Check sheet for the modelled part. Datum: model origin and axes. Units: mm. Face numbers are marked on the shaded views. A direction names the side the tool comes from. Round coordinates to 2 decimals unless told otherwise and drop trailing zeros. Write each loop counter-clockwise with the first axis right and the second up, starting at its lowest first coordinate (ties: lowest second). Pieces come first, ordered by that corner, then holes.
Item 1: Depth check by flat-ended pin: pin 1 (8.5 mm diameter, centred on x = -20, z = -13.5, fed in from -Y); pin 2 (1.4 mm diameter, centred on x = -1.5, z = 24.5, fed in from -Y); pin 3 (1.4 mm diameter, centred on x = 3.5, z = -25, fed in from -Y); pin 4 (23 mm diameter, centred on x = -8, z = 8, fed in from -Y). Enter the tip coordinate at first touch or a pass-through.
Item 2: Section check B-B, the plane z = 0. Record the cut outline in (x, y).
Item 3: Section check C-C, the plane y = 90.5. Record the cut outline in (x, z), plus the area to 3 significant figures.
Item 4: Set-up check for the marked faces 1, 2, 3, 4 and 5: record each of +Z, -Z, +X, -X, +Y, -Y from which the full face is reachable in a straight line by a thin tool's end or side.
Item 5: Material ranges on line 1 along Z through (x, y) = (0, 98); line 2 along Z through (x, y) = (0, 87.75); line 3 along Y through (x, z) = (11, 14.5), recorded low to high.
Item 6: Section check A-A, the plane y = 106. Record the cut outline in (x, z) (3 decimals), plus the area to 3 significant figures.
from build123d import *

# Parameters (mm, degrees)
PAD_DEPTH          = 13
CHAMFER_SIZE       = 2
POLARPATTERN_COUNT = 6
CHAMFER001_SIZE    = 2
CHAMFER002_SIZE    = 2


with BuildPart() as part:
    # Sketch → Revolution (revolve)
    with BuildSketch(Plane.XY):
        Polygon((-11.623481, 80.619493), (-16.623481, 80.619493), (-16.623481, 82.619493), (-22.873481, 82.619493), (-22.873481, 86.619493), (-17.837431, 86.619493), (-17.837431, 91.619493), (-25.337431, 91.619493), (-25.337431, 99.619493), (-12.837431, 99.619493), (-12.837431, 93.119493), (-11.623481, 93.119493), align=None)
    revolve(axis=Axis((0, 0, 0), (0, 1, 0)))

    # Sketch002 (on Face9 of Revolution) → Pad (new body)
    with BuildSketch(Plane(origin=(0, 99.619493, 0), x_dir=(-1, 0, 0), z_dir=(0, 1, 0))):
        with BuildLine():
            Line((3.768044, 12.382216), (7.894003, 24.07634))
            ThreePointArc((7.894003, 24.07634), (0.517974, 25.334484), (-6.903315, 24.378877))
            Line((-3.51886, 12.454993), (-6.903315, 24.378877))
            ThreePointArc((3.768044, 12.382216), (0.129841, 12.944225), (-3.51886, 12.454993))
        make_face()
    pad = extrude(amount=PAD_DEPTH)

    # Chamfer
    chamfer_edges = [part.edges().sort_by_distance(p)[0] for p in [
        (-5.831023, 112.619493, 18.229278),
        (5.211088, 112.619493, 18.416935),
    ]]
    chamfer(chamfer_edges, length=CHAMFER_SIZE)

    # PolarPattern: Pad ×6 about axis
    polarpattern_axis = Axis((0, 99.619493, 0), (0, 1, 0))
    for i in range(1, POLARPATTERN_COUNT):
        add(pad.rotate(polarpattern_axis, i * 360 / POLARPATTERN_COUNT))

    # Chamfer001
    chamfer001_edges = [part.edges().sort_by_distance(p)[0] for p in [
        (18.555078, 112.619493, 4.695533),
        (12.871506, 112.619493, 14.164453),
        (18.702529, 112.619493, -4.064825),
        (13.34399, 112.619493, -13.721402),
        (5.831023, 112.619493, -18.229278),
        (-5.211088, 112.619493, -18.416935),
        (-12.871506, 112.619493, -14.164453),
        (-18.555078, 112.619493, -4.695533),
        (-18.702529, 112.619493, 4.064825),
        (-13.34399, 112.619493, 13.721402),
    ]]
    chamfer(chamfer001_edges, length=CHAMFER001_SIZE)

    # Chamfer002
    chamfer002_edges = [part.edges().sort_by_distance(p)[0] for p in [
        (25.337431, 91.619493, 0),
        (22.873481, 86.619493, 0),
    ]]
    chamfer(chamfer002_edges, length=CHAMFER002_SIZE)


solid = part.part
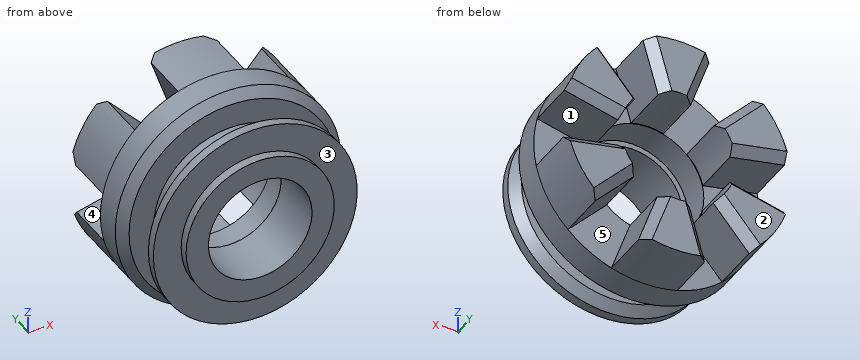
Values found:
1. pin 1: stops at y = 82.62
1. pin 2: stops at y = 92.13
1. pin 3: stops at y = 92.83
1. pin 4: stops at y = 80.62
2. outline: (-25.34, 93.62) - (-23.34, 91.62) - (-17.84, 91.62) - (-17.84, 86.62) - (-20.87, 86.62) - (-22.87, 84.62) - (-22.87, 82.62) - (-16.62, 82.62) - (-16.62, 80.62) - (-11.62, 80.62) - (-11.62, 93.12) - (-12.84, 93.12) - (-12.84, 99.62) - (-25.34, 99.62) - close; (11.62, 80.62) - (16.62, 80.62) - (16.62, 82.62) - (22.87, 82.62) - (22.87, 84.62) - (20.87, 86.62) - (17.84, 86.62) - (17.84, 91.62) - (23.34, 91.62) - (25.34, 93.62) - (25.34, 99.62) - (12.84, 99.62) - (12.84, 93.12) - (11.62, 93.12) - close
3. outline: circle Ø35.67 at (0, 0); hole circle Ø23.25 at (0, 0)
3. area: 575 mm2
4. face 1: +X, +Y
4. face 2: +Z, -Z, +X, -X, +Y
4. face 3: -Y
4. face 4: -X, +Y
4. face 5: +Y
5. line 1: z = -25.34 to -12.84, 12.84 to 25.34
5. line 2: z = -17.84 to -11.62, 11.62 to 17.84
5. line 3: y = 82.62 to 86.62, 91.62 to 99.62
6. outline: (-24.798, 5.202) - (-12.607, 2.928) arc R12.891 cw to (-9.027, 9.275) - (-17.661, 18.168) arc R25.286 ccw to start; (-24.564, -6.211) arc R25.286 ccw to (-16.904, -18.875) - (-8.839, -9.454) arc R12.891 cw to (-12.546, -3.18) - close; (-7.894, 24.076) - (-3.768, 12.382) arc R12.891 cw to (3.519, 12.455) - (6.903, 24.379) arc R25.286 ccw to start; (-6.903, -24.379) arc R25.286 ccw to (7.894, -24.076) - (3.768, -12.382) arc R12.891 cw to (-3.519, -12.455) - close; (8.839, 9.454) arc R12.891 cw to (12.546, 3.18) - (24.564, 6.211) arc R25.286 ccw to (16.904, 18.875) - close; (9.027, -9.275) - (17.661, -18.168) arc R25.286 ccw to (24.798, -5.202) - (12.607, -2.928) arc R12.891 cw to start
6. area: 833 mm2
